from build123d import *

# Parameters (mm, degrees)
ESBO_O2_R                = 1.820066551
ESBO_O2_R_2              = 1.6002
ESBO_O2_R_3              = 1.768261329
RESSALTO_EXTRUS_O1_DEPTH = 1.5
ARQUIVOS_LOCAIS1_R       = 1.5
RESSALTO_EXTRUS_O2_DEPTH = 2.5
ARQUIVOS_LOCAIS2_W       = 12
ARQUIVOS_LOCAIS2_H       = 6.934834447
RESSALTO_EXTRUS_O3_DEPTH = 0.2
ARQUIVOS_LOCAIS3_W       = 21.475999934
ARQUIVOS_LOCAIS3_H       = 29
RESSALTO_EXTRUS_O4_DEPTH = 5.5


with BuildPart() as part:
    # Esboço2 → Ressalto-extrusão1 (new body)
    with BuildSketch(Plane.XY):
        with BuildLine():
            Line((66.770810212, -1.788001123), (66.516852098, -1.788001123))
            ThreePointArc((66.516852098, -1.788001123), (66.067836522, -1.601984783), (65.881852046, -1.152956008))
            Line((65.881852046, -1.152956008), (65.881852046, 11.567000327))
            ThreePointArc((65.881852046, 11.567000327), (66.067868997, 12.016014785), (66.516897161, 12.20199865))
            Line((66.516897161, 12.20199865), (66.770852104, 12.20199865))
            ThreePointArc((66.770852104, 12.20199865), (67.219867652, 12.38801502), (67.405852112, 12.837043786))
            Line((67.405852112, 12.837043786), (67.405852112, 35.941000874))
            ThreePointArc((67.405852112, 35.941000874), (67.107342698, 36.659508424), (66.388413427, 36.957000731))
            Line((66.388413427, 36.957000731), (-34.193146911, 36.957000731))
            ThreePointArc((-34.193146911, 36.957000731), (-34.642164318, 36.770979998), (-34.82814905, 36.321947678))
            Line((-34.82814905, 36.321947678), (-34.82814905, 36.068000792))
            ThreePointArc((-34.82814905, 36.068000792), (-35.014158502, 35.618987038), (-35.463182564, 35.43300247))
            Line((-35.463182564, 35.43300247), (-48.183144777, 35.43300247))
            ThreePointArc((-48.183144777, 35.43300247), (-48.632160998, 35.619010573), (-48.818146915, 36.068035984))
            Line((-48.818146915, 36.068035984), (-48.818146915, 36.322002409))
            ThreePointArc((-48.818146915, 36.322002409), (-49.004168997, 36.771017349), (-49.453199968, 36.957000732))
            Line((-49.453199968, 36.957000732), (-65.563142032, 36.957000732))
            ThreePointArc((-65.563142032, 36.957000732), (-66.281654952, 36.658489436), (-66.57914953, 35.939554956))
            Line((-66.57914953, 35.939554956), (-66.57914953, 18.923000336))
            Line((-66.57914953, 18.923000336), (-69.119142817, 16.38299942))
            Line((-69.119142817, 16.38299942), (-69.119142817, -16.38299942))
            Line((-69.119142817, -16.38299942), (-66.57914953, -18.922999382))
            Line((-66.57914953, -18.922999382), (-66.57914953, -25.526999235))
            ThreePointArc((-66.57914953, -25.526999235), (-66.280636326, -26.245507951), (-65.561704328, -26.543000285))
            Line((-65.561704328, -26.543000285), (66.389851048, -26.543000285))
            ThreePointArc((66.389851048, -26.543000285), (67.108359334, -26.244491656), (67.405852096, -25.525562163))
            Line((67.405852096, -25.525562163), (67.405852096, -2.422999446))
            ThreePointArc((67.405852096, -2.422999446), (67.219837234, -1.973985183), (66.770810212, -1.788001123))
        make_face()
        with Locations((-60.86414892, 19.812000732)):
            Circle(ESBO_O2_R, mode=Mode.SUBTRACT)
        with Locations((-22.76414892, 29.336990572)):
            Circle(ESBO_O2_R_2, mode=Mode.SUBTRACT)
        with Locations((1.36585108, 14.097000732)):
            Circle(ESBO_O2_R_2, mode=Mode.SUBTRACT)
        with Locations((-29.11414892, -18.922999268)):
            Circle(ESBO_O2_R_2, mode=Mode.SUBTRACT)
        with Locations((1.36585108, -13.842999268)):
            Circle(ESBO_O2_R_2, mode=Mode.SUBTRACT)
        with Locations((52.16585108, 29.337000732)):
            Circle(ESBO_O2_R_2, mode=Mode.SUBTRACT)
        with Locations((53.43585108, -18.922999268)):
            Circle(ESBO_O2_R_3, mode=Mode.SUBTRACT)
    extrude(amount=RESSALTO_EXTRUS_O1_DEPTH)

    # Arquivos locais1 → Ressalto-extrusão2 (add)
    with BuildSketch(Plane(origin=(0, 0, 0), x_dir=(-1, 0, 0), z_dir=(0, 0, -1))):
        with Locations((43.07914953, -13.043000285)):
            Circle(ARQUIVOS_LOCAIS1_R)
        with Locations((53.57914953, -13.043000285)):
            Circle(ARQUIVOS_LOCAIS1_R)
        with Locations((43.07914953, -22.043000285)):
            Circle(ARQUIVOS_LOCAIS1_R)
        with Locations((53.57914953, -22.043000285)):
            Circle(ARQUIVOS_LOCAIS1_R)
    extrude(amount=RESSALTO_EXTRUS_O2_DEPTH)

    # Arquivos locais2 → Ressalto-extrusão3 (add)
    with BuildSketch(Plane(origin=(0, 0, 0), x_dir=(-1, 0, 0), z_dir=(0, 0, -1))):
        with Locations((60.57914953, 28.424417956)):
            Rectangle(ARQUIVOS_LOCAIS2_W, ARQUIVOS_LOCAIS2_H)
    extrude(amount=RESSALTO_EXTRUS_O3_DEPTH)

    # Arquivos locais3 → Ressalto-extrusão4 (add)
    with BuildSketch(Plane.XY.offset(1.5)):
        with Locations((55.143852079, 5.20702216)):
            Rectangle(ARQUIVOS_LOCAIS3_W, ARQUIVOS_LOCAIS3_H)
    extrude(amount=RESSALTO_EXTRUS_O4_DEPTH)


solid = part.part
CAD build for the part. Positions are in the model's coordinates, mm. A direction names the side the tool comes from. Give positions to 0.01 mm unless a question says otherwise; leave off trailing zeros. Write each loop counter-clockwise with the first axis right and the second up, starting at its lowest first coordinate (ties: lowest second). Pieces come first, ordered by that corner, then holes. Notation, with made-up numbers: (-37, 41) -> (6, 41) arc R23 ccw to (6, 75) -> close; hole circle Ø11 at (81, -37.75). An arc over 180 degrees is marked (long way). Return JSON: item names as keys, results as strings.
Item 1: Drill centre lines: probe 1 along X at (y, z) = (-20, 1.25); probe 2 along Z at (x, y) = (-35, 0); probe 3 along Y at (x, z) = (54.5, 0.5). Where is each one in solid material? Low to high.
Answer below:
{"probe 1": "x = -66.58 to -30.3, -27.93 to 52.03, 54.84 to 67.41", "probe 2": "z = 0 to 1.5", "probe 3": "y = -26.54 to -20.34, -17.51 to 36.96"}
Item 2: Tool access for faces 1 (the cylindrical face through (-52.39, -13.96, -1.23)), 2 (the flat face through (44.406, 5, 4)), 3 (the cylindrical face through (-24.03, 28.36, 0.74)): list every direction of +Z, -Z, +X, -X, +Y, -Y with a clear straight run to the whole face (end or side of a thin tool).
Answer below:
{"face 1": "-Z", "face 2": "+Z, -X, +Y, -Y", "face 3": "+Z, -Z"}
Item 3: Band-saw the part on C-C (x = -43). List the corners of the cut face in (y, z), then the cut area to 3 significant figures.
Answer below:
{"outline": "(-26.54, 0) -> (-23.54, 0) -> (-23.54, -2.5) -> (-20.55, -2.5) -> (-20.55, 0) -> (-14.54, 0) -> (-14.54, -2.5) -> (-11.55, -2.5) -> (-11.55, 0) -> (35.43, 0) -> (35.43, 1.5) -> (-26.54, 1.5) -> close", "area": "108 mm2"}
Item 4: Band-saw the part on A-A (x = 58). List the corners of the cut face in (y, z).
Answer below:
{"outline": "(-26.54, 0) -> (36.96, 0) -> (36.96, 1.5) -> (19.71, 1.5) -> (19.71, 7) -> (-9.29, 7) -> (-9.29, 1.5) -> (-26.54, 1.5) -> close"}
Item 5: Drop flat-ended pins along their axis: pin 1 (19 mm diameter, centred on x = 13, y = 0, fed in from +Z); pin 2 (19 mm diameter, centred on x = -29, y = 4, fed in from -Z); pin 3 (1.6 mm diameter, centred on x = -41, z = 1, fed in from +Y); pin 4 (1.9 mm diameter, centred on x = 52.17, y = 29.34, fed in from -Z). Give the stop position or say it passes through.
Answer below:
{"pin 1": "stops at z = 1.5", "pin 2": "stops at z = 0", "pin 3": "stops at y = 35.43", "pin 4": "passes through"}
Item 6: Band-saw the part on B-B (z = 4.5). List the corners of the cut face in (x, y), then the cut area to 3 significant figures.
Answer below:
{"outline": "(44.41, -9.29) -> (65.88, -9.29) -> (65.88, 19.71) -> (44.41, 19.71) -> close", "area": "623 mm2"}
Item 7: Two-plate mould, pull along X, no slides. Class faces 4 (the flat face through (-2, 6, 1.5)), 5 (the flat face through (-67.9, -17.6, 0.7)), 6 (the cylindrical face through (-41.58, -12.98, -1.23)): +X half, -X half, draft (parallel to the pull), parting line (faces both ways), or undercut.
Answer below:
{"face 4": "draft", "face 5": "-X half", "face 6": "undercut"}
Item 8: Band-saw the part on D-D (x = -4). List the corners of the cut face in (y, z), then the cut area to 4 significant figures.
Answer below:
{"outline": "(-26.54, 0) -> (36.96, 0) -> (36.96, 1.5) -> (-26.54, 1.5) -> close", "area": "95.25 mm2"}
